Design review of the part shown in the three views and the two pictorial views. Dimensions are in mm from the part's minimum x, y and z. A direction names the side the tool comes from. Give positions to 0.01 mm unless a question says otherwise; leave off trailing zeros. Loops run counter-clockwise (first coordinate to the right, second up) from the corner with the lowest first, then second, coordinate; pieces in that order, holes last. Notation, with made-up numbers: (42.5, 70) - (56.5, 70) arc R22 cw to (56.5, 95) - close; hole circle Ø3 at (57.5, 21). An arc over 180 degrees is marked (long way). Answer as a JSON object with one key per item and string values.
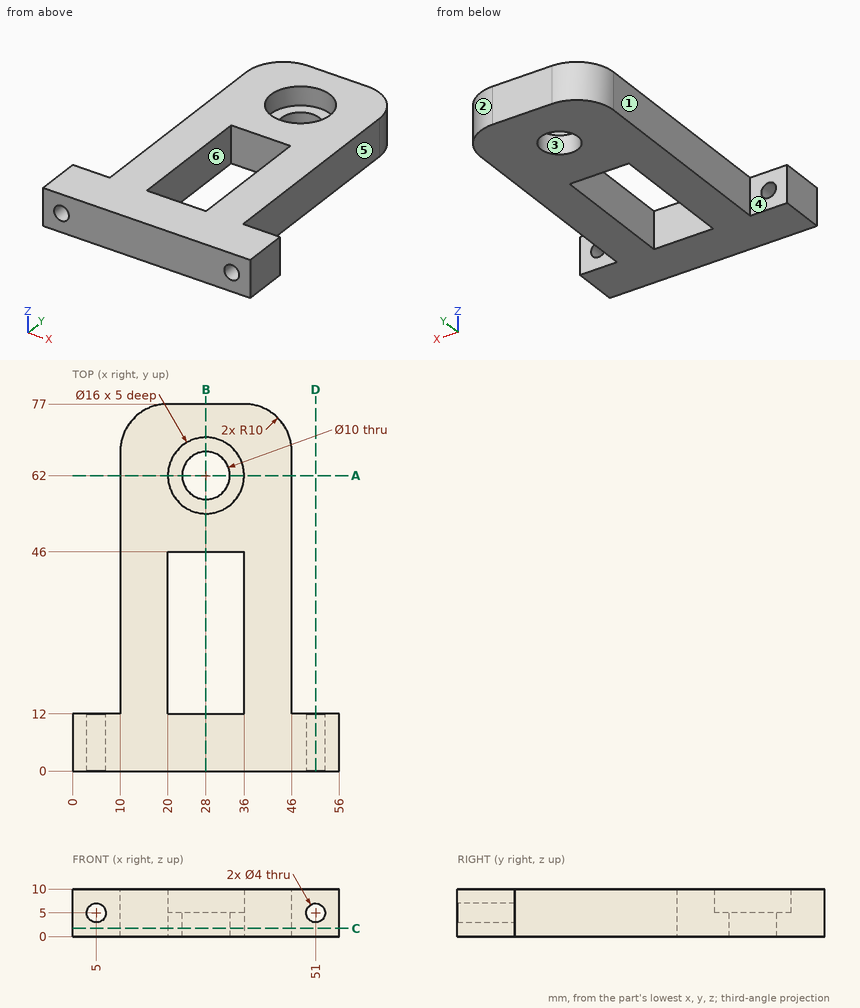
Q1. The part is to be moulded in two halves that separate along Y. For the marked faces 1, 2 and 3, say which applies: +Y half, -Y half, draft (parallel to the pull), parting line (faces both ways), or undercut.
Results:
{"face 1": "draft", "face 2": "+Y half", "face 3": "undercut"}
Q2. Consider section C-C, the plane z = 1.75. State the section outline as (x, y) points.
Results:
{"outline": "(0, 0) - (56, 0) - (56, 12) - (46, 12) - (46, 67) arc R10 ccw to (36, 77) - (20, 77) arc R10 ccw to (10, 67) - (10, 12) - (0, 12) - close; hole (20, 12) - (36, 12) - (36, 46) - (20, 46) - close; hole circle Ø10 at (28, 62)"}
Q3. Consider section B-B, the plane x = 28. State the section outline as (y, z) points.
Results:
{"outline": "(0, 0) - (12, 0) - (12, 10) - (0, 10) - close; (46, 0) - (57, 0) - (57, 5) - (54, 5) - (54, 10) - (46, 10) - close; (67, 0) - (77, 0) - (77, 10) - (70, 10) - (70, 5) - (67, 5) - close"}
Q4. Consider section D-D, the plane x = 51. State the section outline as (y, z) points.
Results:
{"outline": "(0, 0) - (12, 0) - (12, 3) - (0, 3) - close; (0, 7) - (12, 7) - (12, 10) - (0, 10) - close"}
Q5. Clearance check with flat-ended pins moving along their axes: pin 1 Ø4.5 at (x, z) = (5, 5) entering from +Y; pin 2 Ø5 at (y, z) = (26.5, 3.5) entering from -X; pin 3 Ø3 at (y, z) = (23, 4) entering from +X. State where each tip first meets the part, or that it passes through.
Results:
{"pin 1": "stops at y = 12", "pin 2": "stops at x = 10", "pin 3": "stops at x = 46"}
Q6. To check wall thickness, follow probe 1 along Y at (x, z) = (28, 2.2); probe 2 along X at (y, z) = (31.5, 1.5); probe 3 along Y at (x, z) = (22, 1.25). State the ranges of each line that lie inside material, in increasing order. Write a range as [from, to].
Results:
{"probe 1": "y = [0, 12], [46, 57], [67, 77]", "probe 2": "x = [10, 20], [36, 46]", "probe 3": "y = [0, 12], [46, 77]"}
Q7. Consider section A-A, the plane y = 62. State the section outline as (x, z) points.
Results:
{"outline": "(10, 0) - (23, 0) - (23, 5) - (20, 5) - (20, 10) - (10, 10) - close; (33, 0) - (46, 0) - (46, 10) - (36, 10) - (36, 5) - (33, 5) - close"}
Q8. For the marked faces 4, 5 and 6, list the 3-axis set-ups (+Z, -Z, +X, -X, +Y, -Y) from which the entire face can be reached by the end or side of a thin tool; tool diameter is ignored.
Results:
{"face 4": "+Z, -Z, -X, +Y", "face 5": "+Z, -Z, +X, +Y", "face 6": "+Z, -Z"}
